Verification items for the finished model (mm, model axes). Round coordinates to 2 decimals unless told otherwise and drop trailing zeros. Order: outer loops, then holes, each group sorted by start corner. A loop starts at its lowest first (then second) coordinate and runs counter-clockwise, first axis right, second up. Notation, with made-up numbers: (-5, -12.75) -> (29, -12.75) arc R24 ccw to (29, 20.25) -> close; hole circle Ø6 at (22, -27.75). An arc over 180 degrees is marked (long way). Put each result on its own line as item: value.
Autodesk Inventor part; units mm, degrees
ref_plane "YZ Plane" through (0, 0, 0) normal (1, 0, 0) x (0, 1, 0)
ref_plane "XZ Plane" through (0, 0, 0) normal (0, 1, 0) x (-1, 0, 0)
ref_plane "XY Plane" through (0, 0, 0) normal (0, 0, 1) x (1, 0, 0)
sketch "Boceto1" plane through (0, 0, 0) normal (0, 0, 1) x (1, 0, 0)
  line L0 (-25.8, 19.8) -> (25.8, 19.8)
  line L1 (25.8, 19.8) -> (25.8, -19.8)
  line L2 (25.8, -19.8) -> (-25.8, -19.8)
  line L3 (-25.8, -19.8) -> (-25.8, 19.8)
  line L4 (-25.8, 19.8) -> (25.8, -19.8) construction
  line L5 (25.8, 19.8) -> (-25.8, -19.8) construction
  point P0 (0, 0)
  dimension "d0" = 39.6
  dimension "d1" = 51.6
extrude "Extrusión1" add sketch "Boceto1" along normal blind 13
sketch "Boceto2" plane through (0, 0, 13) normal (0, 0, 1) x (1, 0, 0)
  circle A0 centre (-17.9984, 14) radius 2.1
  circle A1 centre (20, 14) radius 2.1
  line L0 (25.8, -19.8) -> (25.8, 19.8)
  line L1 (25.8, 19.8) -> (-25.8, 19.8)
  line L2 (-25.8, 19.8) -> (-25.8, -19.8)
  line L3 (20, 14) -> (-25.8, 14) construction
  line L4 (-25.8, 0) -> (25.8, 0) construction
  circle A2 centre (-17.9984, -14) radius 2.1
  circle A3 centre (20, -14) radius 2.1
  point P0 (0, 0)
  dimension "d4" = 4.2
  dimension "d5" = 4.2
  dimension "d7" = 5.8
  dimension "d8" = 5.8
  dimension "d10" = 5.8
  dimension "d11" = 7.8016
extrude "Extrusión2" cut sketch "Boceto2" against normal through all
properties part number "PiezaNivel" material "Plástico ABS"
Item 1: Section check A-A on y = 14. Record the boundary of the cut face in (x, z), then the cut area to 3 significant figures.
Check sheet entries:
outline: (-25.8, 0) -> (-20.1, 0) -> (-20.1, 13) -> (-25.8, 13) -> close; (-15.9, 0) -> (17.9, 0) -> (17.9, 13) -> (-15.9, 13) -> close; (22.1, 0) -> (25.8, 0) -> (25.8, 13) -> (22.1, 13) -> close
area: 562 mm^2
Item 2: Release check for a two-part mould opening along X. For faces 1 (the flat face through (25.8, 0, 6)), 2 (the flat face through (0, 0, 0)), 3 (the cylindrical face through (-20.096, 14.092, 6.591)), 4 (the flat face through (-25.8, 0, 6)) record: +X half, -X half, draft (parallel to the pull), parting line (faces both ways), or undercut.
Check sheet entries:
face 1: +X half
face 2: draft
face 3: undercut
face 4: -X half
Item 3: Section check B-B on x = 20. Record the boundary of the cut face in (y, z), then the cut area to 3 significant figures.
Check sheet entries:
outline: (-19.8, 0) -> (-16.1, 0) -> (-16.1, 13) -> (-19.8, 13) -> close; (-11.9, 0) -> (11.9, 0) -> (11.9, 13) -> (-11.9, 13) -> close; (16.1, 0) -> (19.8, 0) -> (19.8, 13) -> (16.1, 13) -> close
area: 406 mm^2
Item 4: Section check C-C on z = 11.5. Record the boundary of the cut face in (x, y), then the cut area to 3 significant figures.
Check sheet entries:
outline: (-25.8, -19.8) -> (25.8, -19.8) -> (25.8, 19.8) -> (-25.8, 19.8) -> close; hole circle Ø4.2 at (-18, -14); hole circle Ø4.2 at (-18, 14); hole circle Ø4.2 at (20, -14); hole circle Ø4.2 at (20, 14)
area: 1,990 mm^2
Item 5: Material ranges on L1, parallel to Y at x = -17.5, z = 2; L2, parallel to Y at x = 20, z = 5.75; L3, parallel to X at y = -15, z = 9.75, recorded low to high. Write a range as [from, to].
Check sheet entries:
L1: y = [-19.8, -16.04], [-11.96, 11.96], [16.04, 19.8]
L2: y = [-19.8, -16.1], [-11.9, 11.9], [16.1, 19.8]
L3: x = [-25.8, -19.85], [-16.15, 18.15], [21.85, 25.8]
